The model under review builds one solid part; all positions refer to its coordinate system, in mm. A direction names the side the tool comes from. Give positions to 0.01 mm unless a question says otherwise; leave off trailing zeros. Loops run counter-clockwise (first coordinate to the right, second up) from the corner with the lowest first, then second, coordinate; pieces in that order, holes last. Notation, with made-up numbers: (24, 2.5) -> (31, 2.5) arc R32 cw to (31, 37.5) -> close; hole circle Ø7 at (-20, -34). An arc over 180 degrees is marked (long way). Write each question's results on one line, items separated by ' | '. Start each with the question number.
Q1. We need section C-C (x = -9.75). Write out the cut boundary in (y, z), plus the area to 3 significant figures.
Q2. We need section A-A (z = -58.5). Give the number of separate pieces and of enclosed holes in the cut face, plus the area to 3 significant figures.
Q3. Machinability: for faces 5 (the face through (-11.85, 11, -69)), 6 (the face through (-13, 4.5, -58)), 7 (the face through (12.3, 4.5, -58.4)), 8 (the face through (12.68, 14.61, -27.88)), which of the approach directions +Z, -Z, +X, -X, +Y, -Y give a long, thin tool a straight path to every point of the face, cutting with its end or side? Answer none if there is none.
Q4. We need section D-D (y = 7.75). Write out the cut boundary in (x, z) (3 decimals).
Q5. Wall thickness on L1, parallel to Z at x = -9, y = 14.5; L2, parallel to Z at x = 12.75, y = 12.75; L3, parallel to Y at x = 2.5, z = -66: over which ranges is each line inside the solid? List them lowest first. Write a range as [from, to].
Q6. Mouldability with a two-part tool opening along X and no side actions: class faces 1 (the face through (-14.835, 6, -37)), 2 (the face through (-6.835, 1, -32)), 3 (the face through (14.833, 7, -28)), 4 (the face through (0, 16.75, -31)) as released by +X, released by -X, zero draft, split by the parting line, or undercut.
Q7. Insertion check: pin 1 Ø2 at (x, z) = (-4.5, -20.5) entering from +Y; pin 2 Ø2 at (x, z) = (-11, -57.5) entering from +Y; pin 3 Ø2 at (x, z) = (3, -70) entering from -Y. Each pin has a flat end and moves straight along its axis. Give the tip position at first contact, or say it passes through.
from build123d import *

# Parameters (mm, degrees)
BOSS_EXTRUDE1_DEPTH = 72
BOSS_EXTRUDE3_DEPTH = 5
CUT_EXTRUDE4_DEPTH  = 5
BOSS_EXTRUDE4_DEPTH = 5
BOSS_EXTRUDE5_START = 7
BOSS_EXTRUDE5_DEPTH = 55
CUT_EXTRUDE8_DEPTH  = 5
SKETCH19_W          = 15
SKETCH19_H          = 12.25
BOSS_EXTRUDE8_DEPTH = 7
CUT_EXTRUDE9_REACH  = 78.51
SKETCH20_R          = 1.5
SKETCH21_W          = 23.7
SKETCH21_H          = 22.72285099
CUT_EXTRUDE10_DEPTH = 7


with BuildPart() as part:
    # Sketch1 → Boss-Extrude1 (new body)
    with BuildSketch(Plane.XY):
        Polygon((-14.835, 0), (-6.835, 0), (-6.835, 3), (6.835, 3), (6.835, 0), (14.835, 0), (14.835, 4.5), (8.35, 4.5), (-8.35, 4.5), (-14.835, 4.5), align=None)
    extrude(amount=-BOSS_EXTRUDE1_DEPTH)

    # Sketch8 → Boss-Extrude3 (add)
    with BuildSketch(Plane(origin=(0, 0, -72), x_dir=(-1, 0, 0), z_dir=(0, 0, -1))):
        Polygon((-14.835, 25.70785099), (-14.835, 0), (-10.35, 0), (-10.35, 21.22285099), (10.35, 21.22285099), (10.35, 0), (14.835, 0), (14.835, 25.70785099), align=None)
    extrude(amount=-BOSS_EXTRUDE3_DEPTH)

    # Sketch9 → Cut-Extrude4 (cut)
    with BuildSketch(Plane(origin=(0, 0, -72), x_dir=(-1, 0, 0), z_dir=(0, 0, -1))):
        with BuildLine():
            Line((-15.009070225, 25.881921215), (-15.009070225, 22.527488279))
            ThreePointArc((-15.009070225, 22.527488279), (-13.436955933, 24.309806923), (-11.654637289, 25.881921215))
            Line((-11.654637289, 25.881921215), (-15.009070225, 25.881921215))
        make_face()
        with BuildLine():
            Line((15.009070225, 25.881921215), (15.009070225, 22.527488279))
            ThreePointArc((15.009070225, 22.527488279), (13.436955933, 24.309806923), (11.654637289, 25.881921215))
            Line((11.654637289, 25.881921215), (15.009070225, 25.881921215))
        make_face()
    extrude(amount=-CUT_EXTRUDE4_DEPTH, mode=Mode.SUBTRACT)

    # Sketch11 → Boss-Extrude4 (add)
    with BuildSketch(Plane.XY.offset(-67)):
        with BuildLine():
            Line((14.835, 4.5), (14.835, 22.748275799))
            ThreePointArc((14.835, 22.748275799), (13.436955933, 24.309806923), (11.875424809, 25.70785099))
            Line((11.875424809, 25.70785099), (-11.875424809, 25.70785099))
            ThreePointArc((-11.875424809, 25.70785099), (-13.436955933, 24.309806923), (-14.835, 22.748275799))
            Line((-14.835, 22.748275799), (-14.835, 4.5))
            Line((-14.835, 4.5), (14.835, 4.5))
        make_face()
    extrude(amount=BOSS_EXTRUDE4_DEPTH)

    # Sketch12 → Boss-Extrude5 (add)
    with BuildSketch(Plane.XY.offset(-62).offset(BOSS_EXTRUDE5_START)):
        with BuildLine():
            Line((-14.835, 4.5), (14.832662348, 4.5))
            Line((14.832662348, 4.5), (14.832662348, 9.600169894))
            ThreePointArc((14.832662348, 9.600169894), (12.620742321, 14.666687642), (7.5, 16.75))
            Line((7.5, 16.75), (-7.5, 16.75))
            ThreePointArc((-7.5, 16.75), (-12.68662824, 14.60162824), (-14.835, 9.415))
            Line((-14.835, 9.415), (-14.835, 4.5))
        make_face()
    extrude(amount=BOSS_EXTRUDE5_DEPTH)

    # Sketch18 → Cut-Extrude8 (cut)
    with BuildSketch(Plane(origin=(0, 0, -72), x_dir=(-1, 0, 0), z_dir=(0, 0, -1))):
        Polygon((-10.35, 4.5), (-10.35, 0), (-6.835, 0), (-6.835, 3), (6.835, 3), (6.835, 0), (10.35, 0), (10.35, 4.5), align=None)
    extrude(amount=-CUT_EXTRUDE8_DEPTH, mode=Mode.SUBTRACT)

    # Sketch19 → Boss-Extrude8 (add)
    with BuildSketch(Plane(origin=(0, 0, -55), x_dir=(-1, 0, 0), z_dir=(0, 0, -1))):
        with Locations((0, 10.625)):
            Rectangle(SKETCH19_W, SKETCH19_H)
    extrude(amount=BOSS_EXTRUDE8_DEPTH)

    # Sketch20 → Cut-Extrude9 (cut, up to next)
    with BuildSketch(Plane(origin=(0, 4.5, 0), x_dir=(1, 0, 0), z_dir=(0, 1, 0)), mode=Mode.PRIVATE) as cut_extrude9_sk1:
        with Locations(Location((-10.5425, 58.5, 0), (0, 0, 180))):
            Circle(SKETCH20_R)
    cut_extrude9_tool1 = extrude(cut_extrude9_sk1.sketch, amount=-CUT_EXTRUDE9_REACH, mode=Mode.PRIVATE) & part.part
    # Sketch20 → Cut-Extrude9 (cut, up to next)
    with BuildSketch(Plane(origin=(0, 4.5, 0), x_dir=(1, 0, 0), z_dir=(0, 1, 0)), mode=Mode.PRIVATE) as cut_extrude9_sk2:
        with Locations(Location((10.5425, 58.5, 0), (0, 0, 270))):
            Circle(SKETCH20_R)
    cut_extrude9_tool2 = extrude(cut_extrude9_sk2.sketch, amount=-CUT_EXTRUDE9_REACH, mode=Mode.PRIVATE) & part.part
    add(cut_extrude9_tool1.solids().sort_by_distance((-10.5425, 4.5, -58.5))[0], mode=Mode.SUBTRACT)
    add(cut_extrude9_tool2.solids().sort_by_distance((10.5425, 4.5, -58.5))[0], mode=Mode.SUBTRACT)

    # Sketch21 → Cut-Extrude10 (cut)
    with BuildSketch(Plane(origin=(0, 0, -72), x_dir=(-1, 0, 0), z_dir=(0, 0, -1))):
        with Locations((0, 11.361425495)):
            Rectangle(SKETCH21_W, SKETCH21_H)
    extrude(amount=-CUT_EXTRUDE10_DEPTH, mode=Mode.SUBTRACT)


solid = part.part
Output:
1) outline: (0, -65) -> (22.72, -65) -> (22.72, -72) -> (25.71, -72) -> (25.71, -62) -> (4.5, -62) -> (4.5, -59.77) -> (0, -59.77) -> close; (0, -57.23) -> (4.5, -57.23) -> (4.5, -55) -> (16.4, -55) -> (16.4, 0) -> (0, 0) -> close | area: 1,020 mm2
2) separate pieces: 3 | enclosed holes: 0 | area: 249 mm2
3) face 5: -Z, -Y | face 6: -X, +Y | face 7: +X, +Y | face 8: +Z, +X, +Y
4) outline: (-14.835, -72) -> (-11.85, -72) -> (-11.85, -65) -> (11.85, -65) -> (11.85, -72) -> (14.835, -72) -> (14.835, -62) -> (7.5, -62) -> (7.5, -55) -> (14.833, -55) -> (14.833, 0) -> (-14.835, 0) -> (-14.835, -55) -> (-7.5, -55) -> (-7.5, -62) -> (-14.835, -62) -> close
5) L1: [-65, -62], [-55, 0] | L2: [-72, -62], [-55, 0] | L3: [22.72, 25.71]
6) face 1: released by -X | face 2: undercut | face 3: released by +X | face 4: zero draft
7) pin 1: y = 16.75 | pin 2: y = 4.5 | pin 3: y = 22.72
